Autodesk Fusion 360 part; units mm, degrees
sketch "Sketch1" plane through (0, 0, 0) normal (0, 0, 1) x (1, 0, 0)
  line L0 (-25.4, 38.1) -> (25.4, 38.1)
  line L1 (25.4, 38.1) -> (25.4, -34.29)
  line L2 (25.4, -34.29) -> (-25.4, -34.29)
  line L3 (-25.4, -34.29) -> (-25.4, 38.1)
  dimension "d1" = 50.8
  dimension "d2" = 72.39
extrude "Extrude1" add sketch "Sketch1" along normal blind 7.62
sketch "Sketch2" plane through (0, 0, 0) normal (0, 0, -1) x (1, 0, 0)
  line L0 (25.4, 34.29) -> (-25.4, 34.29)
  line L1 (-25.4, 34.29) -> (-25.4, -38.1)
  line L2 (-25.4, -38.1) -> (25.4, -38.1)
  line L3 (25.4, -38.1) -> (25.4, 34.29)
  circle A0 centre (0, 0) radius 3.937
  dimension "d5" = 7.874
extrude "Extrude2" add sketch "Sketch2" along normal blind 6.985 contours A0
sketch "Sketch3" plane through (0, 0, 7.62) normal (0, 0, 1) x (-1, 0, 0)
  line L0 (25.4, 34.29) -> (-25.4, 34.29)
  line L1 (-25.4, 34.29) -> (-25.4, -38.1)
  line L2 (-25.4, -38.1) -> (25.4, -38.1)
  line L3 (25.4, -38.1) -> (25.4, 34.29)
  line L4 (0, 0) -> (-19.939, 0)
  line L5 (-19.939, 0) -> (-19.939, 29.972)
  line L6 (-19.939, 29.972) -> (19.939, 29.972)
  line L7 (19.939, 29.972) -> (19.939, -30.226)
  line L8 (19.939, -30.226) -> (-19.939, -30.226)
  line L9 (-19.939, -30.226) -> (-19.939, 29.972)
  dimension "d8" = 19.939
  dimension "d9" = 29.972
  dimension "d10" = 39.878
  dimension "d11" = 60.198
extrude "Extrude3" cut sketch "Sketch3" against normal blind 2.54 contours L5 L6 L7 L8 L9
fillet "Fillet1" radius 1.27 4 edges at (19.939, 0.127, 7.62) (0, -29.972, 7.62) (-19.939, 0.127, 7.62) (0, 30.226, 7.62)
fillet "Fillet2" radius 6.35 4 edges at (-25.4, 38.1, 3.81) (-25.4, -34.29, 3.81) (25.4, -34.29, 3.81) (25.4, 38.1, 3.81)
sketch "Sketch4" plane through (0, 0, 5.08) normal (0, 0, 1) x (-1, 0, 0)
  line L0 (-19.939, -30.226) -> (19.939, -30.226)
  line L1 (19.939, -30.226) -> (19.939, 29.972)
  line L2 (19.939, 29.972) -> (-19.939, 29.972)
  line L3 (-19.939, 29.972) -> (-19.939, -30.226)
  line L4 (19.939, -30.226) -> (17.5578, -30.226)
  line L5 (17.5578, -30.226) -> (17.5578, -27.8448)
  line L6 (17.5578, -27.8448) -> (-17.3673, -27.8448)
  line L7 (-17.3673, -27.8448) -> (-17.3673, 26.924)
  line L8 (17.5578, -27.8448) -> (-17.3673, -27.8448)
  line L9 (-17.3673, -27.8448) -> (-17.3673, 26.924)
  line L10 (-17.3673, 26.924) -> (17.5578, 26.924)
  line L11 (17.5578, 26.924) -> (17.5578, -27.8448)
  circle A0 centre (17.5578, 26.924) radius 2.032
  circle A1 centre (17.5578, -27.8448) radius 2.032
  circle A2 centre (-17.3673, -27.8448) radius 2.032
  circle A3 centre (-17.3673, 26.924) radius 2.032
  dimension "d18" = 2.3813
  dimension "d19" = 2.3813
  dimension "d20" = 34.925
  dimension "d21" = 54.7687
  dimension "d22" = 4.064
  dimension "d23" = 4.064
  dimension "d24" = 4.064
  dimension "d25" = 4.064
extrude "Extrude4" add sketch "Sketch4" along normal blind 3.175 contours L5 L6 L8 A1 | L5 L11 A1 | L6 L8 L11 A1 | L6 L7 L8 L9 A2 | L6 L7 L8 L9 A2 | L10 L11 A0 | L10 L11 A0 | L7 L9 L10 A3 | L7 L9 L10 A3
sketch "Sketch5" plane through (0, 0, 8.255) normal (0, 0, 1) x (-1, 0, 0)
  circle A0 centre (17.5578, -27.8448) radius 2.032
  circle A1 centre (17.5578, -27.8448) radius 1.016
  dimension "d28" = 2.032
sketch "Sketch6" plane through (0, 0, 8.255) normal (0, 0, 1) x (-1, 0, 0)
  circle A0 centre (-17.3673, -27.8448) radius 2.032
  circle A1 centre (-17.3673, -27.8448) radius 1.016
  dimension "d29" = 2.032
sketch "Sketch7" plane through (0, 0, 8.255) normal (0, 0, 1) x (-1, 0, 0)
  circle A0 centre (17.5578, 26.924) radius 2.032
  circle A1 centre (17.5578, 26.924) radius 1.016
  dimension "d30" = 2.032
sketch "Sketch8" plane through (0, 0, 8.255) normal (0, 0, 1) x (-1, 0, 0)
  circle A0 centre (-17.3673, 26.924) radius 2.032
  circle A1 centre (-17.3673, 26.924) radius 1.016
  dimension "d31" = 2.032
extrude "Extrude5" cut sketch "Sketch5" sketch "Sketch7" sketch "Sketch6" sketch "Sketch8" against normal blind 5.08 contours A1 of sketch 2 contours A1 of sketch 3 contours A1 of sketch 4 contours A1
fillet "Fillet3" radius 1.27 8 edges at (23.5401, -32.4301, 7.62) (25.4, 1.905, 7.62) (23.5401, 36.2401, 7.62) (0, 38.1, 7.62) (-23.5401, 36.2401, 7.62) (-25.4, 1.905, 7.62) (-23.5401, -32.4301, 7.62) (0, -34.29, 7.62)
equation "d8 = ( 1.57 / 2 ) * 1 in"
equation "d9 = ( 2.36 / 2 ) * 1 in"
equation "d18 = ( 3 / 32 ) * 1 in"
equation "d19 = ( 3 / 32 ) * 1 in"
equation "d26 = ( 1 / 8 ) * 1 in"
The listing builds one solid part. Answer for the finished solid, in the listing's coordinates (mm). A direction names the side the tool comes from. Round coordinates to 2 decimals unless told otherwise and drop trailing zeros. Order: outer loops, then holes, each group sorted by start corner. A loop starts at its lowest first (then second) coordinate and runs counter-clockwise, first axis right, second up. Notation, with made-up numbers: (-18, 26.25) -> (29, 26.25) arc R15 ccw to (29, 46.25) -> close; hole circle Ø5 at (46.5, -10). An arc over 180 degrees is marked (long way). One line per item, written item: value.
Item 1: For a pull along Y with two mould halves and no side action, classify faces 4 (the flat face through (-18, 28, 3.175)), 5 (the flat face through (0, 0, 5.08)), 6 (the flat face through (0, 0, -6.985)), 7 (the cylindrical face through (23.59, 36.19, 3.22)) as released by +Y, released by -Y, zero draft, split by the parting line, or undercut.
Taken from the geometry:
face 4: undercut
face 5: undercut
face 6: zero draft
face 7: released by +Y
Item 2: For faces 1 (the cylindrical face through (-0.853, -3.843, -3.444)), 2 (the flat face through (25.4, 2, 3)), 3 (the cylindrical face through (15.49, 27.07, 6.65)), determine the directions among +Z, -Z, +X, -X, +Y, -Y from which every point of the face is accessible in a straight line to the end or side of a thin tool.
Taken from the geometry:
face 1: -Z
face 2: +Z, -Z, +X, +Y, -Y
face 3: +Z
Item 3: Straight lines are drawn through the part: L1, parallel to X at y = -6, z = 6; L2, parallel to Y at x = 17, z = 5.5; L3, parallel to Z at x = -6, y = -25.5. For each, find the intervals that lie inside material, in ascending order.
Taken from the geometry:
L1: x = -25.4 to -19.94, 19.94 to 25.4
L2: y = -34.29 to -29.97, -28.92 to -27.87, -25.98 to -24.93, 25.85 to 26.9, 28.79 to 29.84, 30.23 to 38.1
L3: z = 0 to 5.08
Item 4: Find section C-C, the plane z = -2.75. Give the vertices of the cut face in (x, y).
Taken from the geometry:
outline: circle Ø7.87 at (0, 0)
Item 5: Find section A-A, the plane x = 0. Give the vertices of the cut face in (y, z) (3 decimals).
Taken from the geometry:
outline: (-34.29, 0) -> (-3.937, 0) -> (-3.937, -6.985) -> (3.937, -6.985) -> (3.937, 0) -> (38.1, 0) -> (38.1, 6.35) arc R1.27 ccw to (36.83, 7.62) -> (31.496, 7.62) arc R1.27 ccw to (30.226, 6.35) -> (30.226, 5.08) -> (-29.972, 5.08) -> (-29.972, 6.35) arc R1.27 ccw to (-31.242, 7.62) -> (-33.02, 7.62) arc R1.27 ccw to (-34.29, 6.35) -> close
Item 6: Find section B-B, the plane y = 0. Give the vertices of the cut face in (x, z) (3 decimals), then the cut area to 3 significant figures.
Taken from the geometry:
outline: (-25.4, 0) -> (-3.937, 0) -> (-3.937, -6.985) -> (3.937, -6.985) -> (3.937, 0) -> (25.4, 0) -> (25.4, 6.35) arc R1.27 ccw to (24.13, 7.62) -> (21.209, 7.62) arc R1.27 ccw to (19.939, 6.35) -> (19.939, 5.08) -> (-19.939, 5.08) -> (-19.939, 6.35) arc R1.27 ccw to (-21.209, 7.62) -> (-24.13, 7.62) arc R1.27 ccw to (-25.4, 6.35) -> close
area: 339 mm2
Item 7: Find section D-D, the plane x = 9. Give the vertices of the cut face in (y, z), then the cut area to 3 significant figures.
Taken from the geometry:
outline: (-34.29, 0) -> (38.1, 0) -> (38.1, 6.35) arc R1.27 ccw to (36.83, 7.62) -> (31.5, 7.62) arc R1.27 ccw to (30.23, 6.35) -> (30.23, 5.08) -> (-29.97, 5.08) -> (-29.97, 6.35) arc R1.27 ccw to (-31.24, 7.62) -> (-33.02, 7.62) arc R1.27 ccw to (-34.29, 6.35) -> close
area: 397 mm2
Item 8: Given P1, Ø1.2, axis at x = 17.37, y = 27.84, coming from the -Z side; P2, Ø1.6, axis at x = -17.56, y = -26.92, coming from the +Z side (3 decimals); P3, Ø5, axis at x = 16.5, y = -15.5, coming from the +Z side, each flat-ended and moving along its own axis, determine where each tip first touches the part or whether it passes through.
Taken from the geometry:
P1: stops at z = 0
P2: stops at z = 3.175
P3: stops at z = 5.08
